Geometry: final body of the model. Coordinates: model frame, mm. A direction names the side the tool comes from. Give positions to 0.01 mm unless a question says otherwise; leave off trailing zeros. Write each loop counter-clockwise with the first axis right and the second up, starting at its lowest first coordinate (ties: lowest second). Pieces come first, ordered by that corner, then holes.
Autodesk Inventor part; units mm, degrees
ref_plane "Work Plane2" through (2.032, 0, 0) normal (0, 1, 0) x (1, 0, 0)
ref_plane "YZ Plane" through (0, 0, 0) normal (1, 0, 0) x (0, 1, 0)
ref_plane "XZ Plane" through (0, 0, 0) normal (0, 1, 0) x (-1, 0, 0)
sketch "Sketch1" plane through (0, 0, 0) normal (0, 0, 1) x (1, 0, 0)
  line L0 (2.2606, 0) -> (9.525, 0)
  line L1 (9.525, 0) -> (9.525, 1.4224)
  line L2 (9.525, 1.4224) -> (1.7018, 1.4224)
  line L3 (0.4892, 2.4765) -> (0, 2.4765)
  line L4 (-1.905, 0) -> (11.43, 0)
  line L5 (0, -0.4953) -> (0, 2.9718)
  line L6 (0, 1.6256) -> (1.8999, 0.6783)
  line L7 (1.8999, 0.6783) -> (2.2606, 0)
  line L8 (1.7018, 1.4224) -> (0.4892, 2.4765)
  line L9 (0, 2.4765) -> (0, 1.6256)
  dimension "d2" = 2.8448
  dimension "d3" = 4.953
  dimension "d4" = 2.2606
  dimension "d5" = 3.2512
  dimension "d6" = 26.5
  dimension "d7" = 62
  dimension "d13" = 41
  dimension "d14" = 1.7018
  dimension "d15" = 9.525
revolve "Body" add sketch "Sketch1" angle 360 about axis through (2.2606, 0, 0) along (1, 0, 0) contours L7 L6 L5 L3 L8 L2 L1 L0
sketch "Sketch2" plane through (0, 0, 0) normal (-1, 0, 0) x (0, 0, 1)
  line L0 (0, -3.4671) -> (0, 3.4671)
  line L1 (-3.4671, 0) -> (3.4671, 0)
  line L2 (0, 1.6256) -> (0, 0) construction
  line L3 (0, 0) -> (1.6256, 0) construction
  arc A0 (0.5419, 0) -> (0, 0.5419) centre (0, 0) ccw
  line L4 (0, 0) -> (0.7947, 0.7947) construction
  arc A1 (0.8128, 0) -> (0, 0.8128) centre (0, 0) ccw construction
  line L5 (0.2286, 1.6094) -> (0.2202, 0.7824)
  line L6 (1.6094, 0.2286) -> (0.7824, 0.2202)
  arc A2 (0.2202, 0.7824) -> (0.7824, 0.2202) centre (0.7767, 0.7767) ccw
  arc A3 (1.6256, 0) -> (1.6094, 0.2286) centre (0, 0) ccw
  arc A4 (0.2286, 1.6094) -> (0, 1.6256) centre (0, 0) ccw
  arc A5 (1.6094, 0.2286) -> (0.2286, 1.6094) centre (0, 0) ccw
  line L7 (0.2286, -1.6094) -> (0.2202, -0.7824)
  line L8 (1.6094, -0.2286) -> (0.7824, -0.2202)
  arc A6 (0.7824, -0.2202) -> (0.2202, -0.7824) centre (0.7767, -0.7767) ccw
  arc A7 (1.6094, -0.2286) -> (1.6256, 0) centre (0, 0) ccw
  arc A8 (0, -1.6256) -> (0.2286, -1.6094) centre (0, 0) ccw
  arc A9 (0.2286, -1.6094) -> (1.6094, -0.2286) centre (0, 0) ccw
  line L9 (-0.2286, 1.6094) -> (-0.2202, 0.7824)
  line L10 (-1.6094, 0.2286) -> (-0.7824, 0.2202)
  arc A10 (-0.7824, 0.2202) -> (-0.2202, 0.7824) centre (-0.7767, 0.7767) ccw
  arc A11 (-1.6094, 0.2286) -> (-1.6256, 0) centre (0, 0) ccw
  arc A12 (0, 1.6256) -> (-0.2286, 1.6094) centre (0, 0) ccw
  arc A13 (-0.2286, 1.6094) -> (-1.6094, 0.2286) centre (0, 0) ccw
  arc A14 (-1.6094, -0.2286) -> (-0.2286, -1.6094) centre (0, 0) ccw
  arc A15 (-0.2286, -1.6094) -> (0, -1.6256) centre (0, 0) ccw
  arc A16 (-1.6256, 0) -> (-1.6094, -0.2286) centre (0, 0) ccw
  line L11 (-1.6094, -0.2286) -> (-0.7824, -0.2202)
  arc A17 (-0.2202, -0.7824) -> (-0.7824, -0.2202) centre (-0.7767, -0.7767) ccw
  line L12 (-0.2286, -1.6094) -> (-0.2202, -0.7824)
  dimension "d18" = 45
  dimension "d19" = 1.0837
  dimension "d20" = 1.6256
  dimension "d21" = 3.2512
  dimension "d22" = 0.2286
extrude "Slot" add sketch "Sketch2" against normal up to next contours A2 L5 A5 L6 | L9 A10 L10 A13 | L7 A6 L8 A9 | A14 L11 A17 L12
fillet "Fillet1" radius 0.0914 4 edges at (0, 1.6256, 0) (0, 0, 1.6256) (0, -1.6256, 0) (0, 0, -1.6256)
thread "Thread"
chamfer "Chamfer1" distance 0.4763 distance2 0.4763 1 edges at (9.525, -1.4224, 0) measured on face at (9.525, 0.2736, 0.8712)
ref_plane "Work Plane2" through (2.032, 0, 0) normal (0, 1, 0) x (1, 0, 0)
equation "\"d2\" = GD"
equation "\"d3\" = KOD"
equation "\"d4\" = INTI"
equation "\"d5\" = SDM"
equation "\"d13\" = 0.5 * SEWI"
equation "\"d14\" = KOH"
equation "\"d15\" = NLG"
equation "\"d19\" = 0.333333 * SDM"
equation "\"d20\" = 0.5 * SDM"
equation "\"d21\" = SDM"
equation "\"d22\" = 0.5 * SBR"
equation "\"d45\" = INTI"
equation "\"d25\" = 0.2 * SBR"
equation "\"d9\" = GEL"
equation "\"d11\" = -0.5 * SPD + 0.5 * GD"
equation "\"d12\" = GUL"
equation "\"GD\" = NND"
equation "\"NLG\" = 9.525"
equation "\"GEL\" = 6.2357"
equation "\"KOD\" = 4.953"
equation "\"KOH\" = 1.7018"
equation "\"SDM\" = 3.2512"
equation "\"INTI\" = 2.2606"
equation "\"SBR\" = 0.4572"
equation "\"GUL\" = 0.75 * GAL"
equation "\"SPD\" = 1.8923"
equation "\"SEWI\" = 82deg"
equation "\"d0\" = NLG"
equation "\"d1\" = KOH"
equation "\"d17\" = SDM"
equation "\"TOA\" = 30deg"
equation "\"THREADDIA\" = 2.8448"
equation "\"BDM\" = NND"
equation "\"NND\" = 2.8448"
equation "\"GAL\" = 0.635"
equation "\"GD1\" = SPD"
properties part number "ANSI B18.6.3 - 4-40 x 3/8, CRFCHMSTII(5)" material "Steel, Mild"
Item 1: Pull-direction query (Y, two-part tool) for faces 3 (the face through (1.17, -1.04, -0.01)), 4 (the face through (9.525, 0, 0)), 5 (the face through (0.241, -0.322, -2.455)); classes: +Y half, -Y half, draft (parallel to the pull), parting line (faces both ways), or undercut.
Found:
face 3: undercut
face 4: draft
face 5: parting line
Item 2: Reachability of faces 1 (the face through (1.17, -0.01, 1.04)), 2 (the face through (5.32, -0.31, 1.39)) from +Z, -Z, +X, -X, +Y, -Y: full face, straight path, thin tool, end or side. Return the list, or none.
Found:
face 1: -X
face 2: +X
Item 3: Section A-A, the plane x = 8. Return the cut outline in (y, z), plus the area to 3 significant figures.
Found:
outline: circle Ø2.84 at (0, 0)
area: 6.36 mm2
Item 4: Line query: L1, parallel to Y at x = 5.25, z = 1.25; L2, parallel to Z at x = 1.5, y = -0.7; L3, parallel to Z at x = 3.5, y = -0.5. Output: solid intervals per line, ascending.
Found:
L1: y = -0.68 to 0.68
L2: z = -1.44 to -0.23, 0.23 to 1.44
L3: z = -1.33 to 1.33
Item 5: Pin query (flat end, axial travel): pin 1 Ø1 at (x, z) = (4, -0.5) entering from +Y; pin 2 Ø1 at (x, y) = (5, -1.5) entering from +Z; pin 3 Ø1 at (y, z) = (2, 0.5) entering from +X. Return the tip coordinate at first contact, or that it passes through.
Found:
pin 1: stops at y = 1.42
pin 2: stops at z = 1.01
pin 3: stops at x = 1.54
